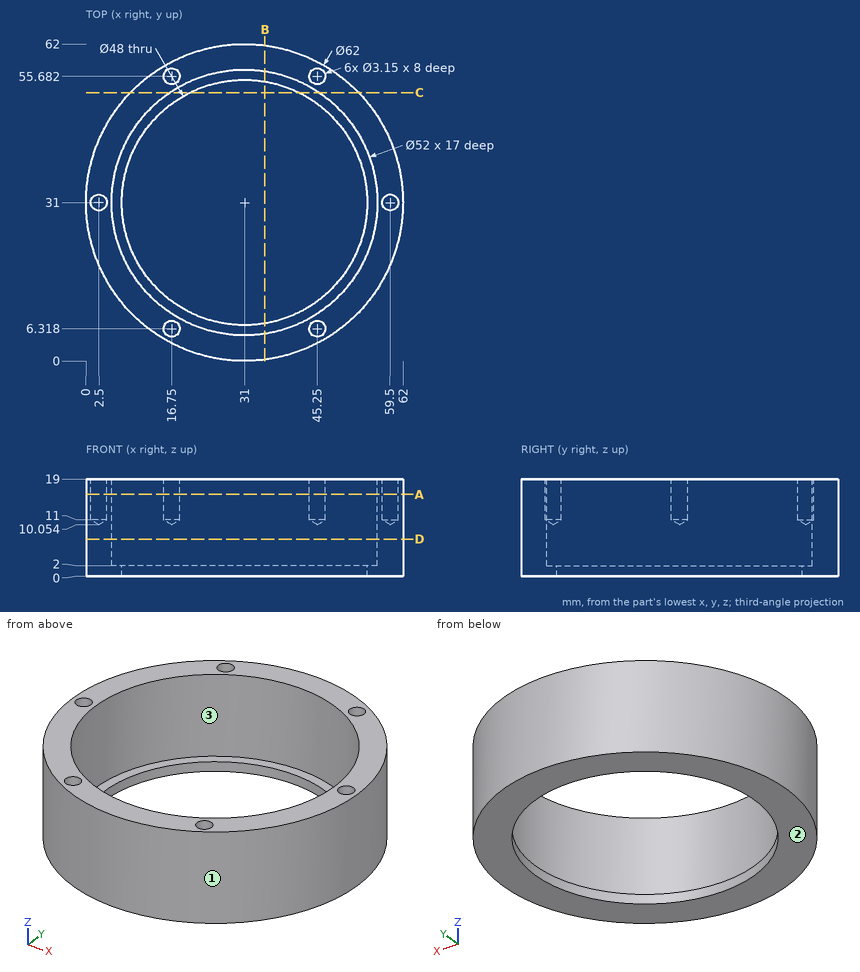
Geometry check sheet. Reference: drawing and pictorial views, mm from the part's lowest x, y, z. Round coordinates to 2 decimals unless told otherwise and drop trailing zeros. Order: outer loops, then holes, each group sorted by start corner. A loop starts at its lowest first (then second) coordinate and runs counter-clockwise, first axis right, second up. Notation, with made-up numbers: M -7,18.5 L 39,18.5 A16 cw 39,48.5 Z; hole C -3.75,77 d11. An arc over 180 degrees is marked long. One line per item, written item: value. Start each with the question number.
1. Release check for a two-part mould opening along X. For the marked faces 1, 2 and 3 record: released by +X, released by -X, zero draft, split by the parting line, or undercut.
2. Scan lines: line 1 along Y through (x, z) = (31.5, 17.5) (1 decimal); line 2 along Z through (x, y) = (54, 41); line 3 along X through (y, z) = (36, 3.5) (1 decimal). Record each from-to range of solid material in increasing order.
3. Section check A-A on z = 16. Give the number of separate pieces and of enclosed holes in the cut face.
4. Section check C-C on y = 52.5. Enter the section's corners in (x, z) (1 decimal).
5. Section check B-B on x = 35. Enter the section's corners in (y, z) (1 decimal).
6. Gauge pin test, flat ends, axial feed: P1, Ø2.5, axis at x = 2.5, y = 31, coming from the +Z side (1 decimal); P2, Ø1.5, axis at x = 39, z = 10.5, coming from the -Y side; P3, Ø1, axis at y = 27.5, z = 11, coming from the -X side. Record the tip position at first contact, or that the pin passes through.
7. Section check D-D on z = 7.25. Enter the section's corners in (x, y).
Results found:
1. face 1: split by the parting line
1. face 2: zero draft
1. face 3: undercut
2. line 1: 0 to 5, 57 to 62
2. line 2: 0 to 2
2. line 3: 0.4 to 5.5, 56.5 to 61.6
3. separate pieces: 1
3. enclosed holes: 7
4. outline: M 8.7,0 L 20.3,0 L 20.3,2 L 16.4,2 L 16.4,19 L 8.7,19 Z; M 41.7,0 L 53.3,0 L 53.3,19 L 45.6,19 L 45.6,2 L 41.7,2 Z
5. outline: M 0.3,0 L 7.3,0 L 7.3,2 L 5.3,2 L 5.3,19 L 0.3,19 Z; M 54.7,0 L 61.7,0 L 61.7,19 L 56.7,19 L 56.7,2 L 54.7,2 Z
6. P1: z = 10.8
6. P2: y = 0.86
6. P3: x = 0.15
7. outline: C 31,31 d62; hole C 31,31 d52
